CAD build for the part. Positions are in the model's coordinates, mm. A direction names the side the tool comes from. Give positions to 0.01 mm unless a question says otherwise; leave off trailing zeros. Loops run counter-clockwise (first coordinate to the right, second up) from the corner with the lowest first, then second, coordinate; pieces in that order, holes last.
Item 1: Drop flat-ended pins along their axis: P1, Ø0.9, axis at x = -1.5, z = 2, coming from the -Y side; P2, Ø3, axis at y = -14.5, z = -2, coming from the -X side; P3, Ø4, axis at x = -7, z = -3, coming from the +Y side. Give the stop position or say it passes through.
Item 2: Mould opens along Z. For faces 1 (the flat face through (-4, -3.439, 6)), 2 (the flat face through (-4.696, -3.833, 3.773)), 3 (the cylindrical face through (-3.015, -11.969, -0.74)), 4 (the cylindrical face through (-1.282, -6.373, 7.378)) say: released by +Z, released by -Z, zero draft, split by the parting line, or undercut.
Item 3: Probe probe 1 along X at (y, z) = (-13, 4.25); probe 2 along Y at (x, z) = (-3.5, 7); probe 3 along Z at (x, y) = (-6.5, -4.5). List the from-to ranges inside material, lowest first.
Item 4: Which spindle directions (+Z, -Z, +X, -X, +Y, -Y) get a long thin tool onto all of the face, cutting with end or side? Do faces 5 (the flat face through (-2, -11.2, 0)), 6 (the cylindrical face through (-7.947, -6.271, 0.692)), 7 (the cylindrical face through (-3.877, -17.411, 1.615)), 8 (the flat face through (-4.6, -5.439, 0.2)). Say none if no direction does.
Item 5: Saw through at B-B on y = -14.5. Give the cut face in (x, z), plus the area to 3 significant figures.
Item 6: Saw through at A-A on z = 4.75. Give the cut face in (x, y).
Item 7: Saw through at C-C on z = -4.5. Give the cut face in (x, y).
from build123d import *

# Parameters (mm, degrees)
ESQUISSE1_W             = 8
ESQUISSE1_H             = 8
EXTRUSION1_DEPTH        = 8
ESQUISSE2_R             = 7.864437578
ESQUISSE2_R_2           = 5.656854249
ENL_V_MAT_EXTRU_1_DEPTH = 9
ESQUISSE3_R             = 8.352248068
ESQUISSE3_R_2           = 5.656854249
ENL_V_MAT_EXTRU_2_DEPTH = 9
EXTRUSION2_DEPTH        = 2
ESQUISSE5_R             = 4
EXTRUSION3_DEPTH        = 2
ESQUISSE6_R             = 2.5
EXTRUSION4_DEPTH        = 4
ESQUISSE7_R             = 3
EXTRUSION5_DEPTH        = 1.5
ESQUISSE8_R             = 4.25
EXTRUSION6_DEPTH        = 6.5
CONG_1_R                = 1
ENL_V_MAT_EXTRU_3_DEPTH = 0.8


with BuildPart() as part:
    # Esquisse1 → Extrusion1 (new body)
    with BuildSketch(Plane.XY):
        with Locations((-4.627553444, -9.439073634)):
            Rectangle(ESQUISSE1_W, ESQUISSE1_H)
    extrude(amount=EXTRUSION1_DEPTH)

    # Esquisse2 → Enlèv. mat.-Extru.1 (cut, symmetric)
    with BuildSketch(Plane(origin=(-4.313776722, 0, 4.313776722), x_dir=(-0.7071067811865488, 0, -0.7071067811865462), z_dir=(0.7071067811865462, 0, -0.7071067811865488))):
        with Locations((0.443747296, -9.439073634)):
            Circle(ESQUISSE2_R)
        with Locations((0.443747296, -9.439073634)):
            Circle(ESQUISSE2_R_2, mode=Mode.SUBTRACT)
    extrude(amount=ENL_V_MAT_EXTRU_1_DEPTH, both=True, mode=Mode.SUBTRACT)

    # Esquisse3 → Enlèv. mat.-Extru.2 (cut, symmetric)
    with BuildSketch(Plane(origin=(-0.313776722, 0, -0.313776722), x_dir=(0.7071067811865483, 0, -0.7071067811865468), z_dir=(0.7071067811865468, 0, 0.7071067811865483))):
        with Locations((-6.100601545, -9.439073634)):
            Circle(ESQUISSE3_R)
        with Locations((-6.100601545, -9.439073634)):
            Circle(ESQUISSE3_R_2, mode=Mode.SUBTRACT)
    extrude(amount=ENL_V_MAT_EXTRU_2_DEPTH, both=True, mode=Mode.SUBTRACT)

    # Esquisse4 → Extrusion2 (add)
    with BuildSketch(Plane(origin=(0, -5.439073634, 0), x_dir=(-1, 0, 0), z_dir=(0, 1, 0))):
        Polygon((2.690239828, 7.546850615), (0.5872339, 4.095662501), (2.524547516, 0.548811886), (6.564867061, 0.453149385), (8.667872988, 3.904337499), (6.730559372, 7.451188114), align=None)
    extrude(amount=EXTRUSION2_DEPTH)

    # Esquisse5 → Extrusion3 (add)
    with BuildSketch(Plane.XZ.offset(13.439073634)):
        with Locations(Location((-4.627553444, 4, 0), (0, 0, 270))):
            Circle(ESQUISSE5_R)
    extrude(amount=EXTRUSION3_DEPTH)

    # Esquisse6 → Extrusion4 (add)
    with BuildSketch(Plane.XZ.offset(15.439073634)):
        with Locations(Location((-4.627553444, 4, 0), (0, 0, 270))):
            Circle(ESQUISSE6_R)
    extrude(amount=EXTRUSION4_DEPTH)

    # Esquisse7 → Extrusion5 (add)
    with BuildSketch(Plane(origin=(0, 0, 0), x_dir=(-1, 0, 0), z_dir=(0, 0, -1))):
        with Locations(Location((4.627553444, -9.439073634, 0), (0, 0, 180))):
            Circle(ESQUISSE7_R)
    extrude(amount=EXTRUSION5_DEPTH)

    # Esquisse8 → Extrusion6 (add)
    with BuildSketch(Plane(origin=(0, 0, -1.5), x_dir=(-1, 0, 0), z_dir=(0, 0, -1))):
        with Locations(Location((4.627553444, -9.439073634, 0), (0, 0, 180))):
            Circle(ESQUISSE8_R)
    extrude(amount=EXTRUSION6_DEPTH)

    # Congé1
    cong_1_edges = [part.edges().sort_by_distance(p)[0] for p in [
        (-8.877553444, -9.439073634, -8),
    ]]
    fillet(cong_1_edges, radius=CONG_1_R)

    # Esquisse9 → Enlèv. mat.-Extru.3 (cut)
    with BuildSketch(Plane(origin=(0, -3.439073634, 0), x_dir=(-1, 0, 0), z_dir=(0, 1, 0))):
        Polygon((1.321943124, 1.93003998), (8.151603046, 5.660446078), (7.960645286, 6.010053204), (1.130985365, 2.279647106), align=None)
    extrude(amount=-ENL_V_MAT_EXTRU_3_DEPTH, mode=Mode.SUBTRACT)


solid = part.part
Results below:
1. P1: stops at y = -15.44
1. P2: stops at x = -6.95
1. P3: stops at y = -5.21
2. face 1: zero draft
2. face 2: undercut
2. face 3: undercut
2. face 4: released by +Z
3. probe 1: x = -8.63 to -0.63
3. probe 2: y = -15.44 to -3.44
3. probe 3: z = 0.45 to 7.46
4. face 5: none
4. face 6: -X, +Y
4. face 7: -Y
4. face 8: +Y
5. outline: circle Ø8 at (-4.63, 4)
5. area: 50.3 mm2
6. outline: (-8.63, -13.44) - (-8.56, -13.44) - (-8.56, -15.44) - (-7.01, -15.44) - (-7.01, -19.44) - (-2.24, -19.44) - (-2.24, -15.44) - (-0.7, -15.44) - (-0.7, -13.44) - (-0.63, -13.44) - (-0.63, -5.44) - (-0.99, -5.44) - (-0.99, -3.44) - (-5.65, -3.44) - (-5.65, -4.24) - (-6.48, -4.24) - (-6.48, -3.44) - (-8.21, -3.44) - (-8.21, -5.44) - (-8.63, -5.44) - close
7. outline: circle Ø8.5 at (-4.63, -9.44)
